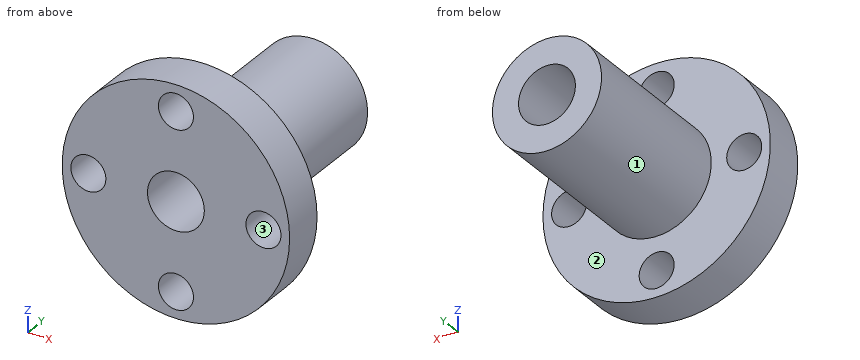
from build123d import *

# Parameters (mm, degrees)
SKETCH1_R           = 12.7
SKETCH1_R_2         = 6.096
SKETCH1_R_3         = 1.9558
SKETCH1_R_4         = 3.175
BOSS_EXTRUDE1_DEPTH = 4.7625
SKETCH1_3_R         = 6.096
SKETCH1_3_R_2       = 3.175
BOSS_EXTRUDE2_DEPTH = 19.05


with BuildPart() as part:
    # Sketch1 → Boss-Extrude1 (new body)
    with BuildSketch(Plane(origin=(0, 0, 0), x_dir=(1, 0, 0), z_dir=(0, 1, 0))):
        Circle(SKETCH1_R)
        Circle(SKETCH1_R_2, mode=Mode.SUBTRACT)
        with Locations((-9.779, 0)):
            Circle(SKETCH1_R_3, mode=Mode.SUBTRACT)
        with Locations((0, -9.779)):
            Circle(SKETCH1_R_3, mode=Mode.SUBTRACT)
        with Locations((9.779, 0)):
            Circle(SKETCH1_R_3, mode=Mode.SUBTRACT)
        with Locations((0, 9.779)):
            Circle(SKETCH1_R_3, mode=Mode.SUBTRACT)
        Circle(SKETCH1_R_2)
        Circle(SKETCH1_R_4, mode=Mode.SUBTRACT)
    extrude(amount=-BOSS_EXTRUDE1_DEPTH)

    # Sketch1_3 → Boss-Extrude2 (add)
    with BuildSketch(Plane(origin=(0, 0, 0), x_dir=(1, 0, 0), z_dir=(0, 1, 0))):
        Circle(SKETCH1_3_R)
        Circle(SKETCH1_3_R_2, mode=Mode.SUBTRACT)
    extrude(amount=BOSS_EXTRUDE2_DEPTH)


solid = part.part
Verification items for the finished model (mm, model axes). Face numbers are marked on the shaded views. Coordinates: 2 decimals unless noted, no trailing zeros. Write each loop counter-clockwise with the first axis right and the second up, starting at its lowest first coordinate (ties: lowest second). Pieces come first, ordered by that corner, then holes. Notation, with made-up numbers: (63, 31) - (120, 31) arc R18 cw to (120, 58) - close; hole circle Ø3 at (50.25, 58). An arc over 180 degrees is marked (long way). Answer as a JSON object with one key per item and string values.
(1) Cross-section at C-C on z = 8.5. Record the cut outline in (x, y), plus the area to 3 significant figures.
Report:
{"outline": "(-9.44, -4.76) - (-1.48, -4.76) - (-1.48, 0) - (-9.44, 0) - close; (1.48, -4.76) - (9.44, -4.76) - (9.44, 0) - (1.48, 0) - close", "area": "75.8 mm^2"}
(2) Thickness scan on line 1 along Z through (x, y) = (0, -3.45) (3 decimals); line 2 along X through (y, z) = (2.75, 0) (3 decimals). Record the ranges inside material, lowest first.
Report:
{"line 1": "-12.7 to -11.735, -7.823 to -3.175, 3.175 to 7.823, 11.735 to 12.7", "line 2": "-6.096 to -3.175, 3.175 to 6.096"}
(3) Cross-section at A-A on z = 0. Give the number of separate pieces and of enclosed holes in the cut face, plus the area to 3 significant figures.
Report:
{"separate pieces": "4", "enclosed holes": "0", "area": "165 mm^2"}
(4) Mould release check, pull along X, two halves, no side actions. Record for the marked faces 1, 2 and 3: pulls with the +X half, pulls with the -X half, needs draft (parallel to the pull), parting line crosses it, or undercut.
Report:
{"face 1": "parting line crosses it", "face 2": "needs draft", "face 3": "undercut"}
(5) Gauge pin test, flat ends, axial feed: pin 1 Ø8 at (x, z) = (4.5, -9.5) entering from +Y; pin 2 Ø5 at (x, y) = (-3, -1.5) entering from -Z; pin 3 Ø6 at (y, z) = (6, -6.5) entering from -X; pin 4 Ø2 at (x, y) = (-8.5, 14) entering from +Z. Record the tip position at first contact, or that the pin passes through.
Report:
{"pin 1": "y = 0", "pin 2": "z = -12.69", "pin 3": "x = -4.99", "pin 4": "through"}
(6) Cross-section at D-D on x = -9. Record the cut outline in (y, z), plus the area to 3 significant figures.
Report:
{"outline": "(-4.76, -8.96) - (0, -8.96) - (0, -1.79) - (-4.76, -1.79) - close; (-4.76, 1.79) - (0, 1.79) - (0, 8.96) - (-4.76, 8.96) - close", "area": "68.3 mm^2"}
